Geometry check sheet. Reference: the model listing, model coordinates, mm. Face numbers are marked on the shaded views. Round coordinates to 2 decimals unless told otherwise and drop trailing zeros. Order: outer loops, then holes, each group sorted by start corner. A loop starts at its lowest first (then second) coordinate and runs counter-clockwise, first axis right, second up. Notation, with made-up numbers: (80, -7.5) - (124, -7.5) arc R29 ccw to (124, 31.5) - close; hole circle Ø7 at (17.25, 16). An arc over 180 degrees is marked (long way). Use a Markdown table: item, result. Add a question column.
(1) Mould release check, pull along Z, two halves, no side actions. Record for the marked faces 1 and 2: released by +Z, released by -Z, zero draft, split by the parting line, or undercut.
(2) Thickness scan on line 1 along Y through (x, z) = (-17, 0); line 2 along Y through (x, z) = (-42.5, 0). Record the ranges inside material, lowest first. Write a range as [from, to].
(3) Section check C-C on x = 18. Record the boundary of the cut face in (y, z), then the cut area to 3 significant figures.
(4) Section check A-A on z = 0. Record the boundary of the cut face in (x, y), then the cut area to 3 significant figures.
(5) Gauge pin test, flat ends, axial feed: P1, Ø4, axis at x = 34, y = -60.5, coming from the +Z side; P2, Ø10, axis at y = -22, z = 0, coming from the -X side; P3, Ø1, axis at y = -40, z = -28.5, coming from the -X side. Record the tip position at first contact, or that the pin passes through.
(6) Section check D-D on y = 68. Record the boundary of the cut face in (x, z).
Autodesk Inventor part; units mm, degrees
ref_plane "YZ Plane" through (0, 0, 0) normal (1, 0, 0) x (0, 1, 0)
ref_plane "XZ Plane" through (0, 0, 0) normal (0, 1, 0) x (-1, 0, 0)
ref_plane "XY Plane" through (0, 0, 0) normal (0, 0, 1) x (1, 0, 0)
sketch "Sketch1" plane through (0, 0, 0) normal (1, 0, 0) x (0, 1, 0)
  arc A0 (0, -80) -> (0, 80) centre (0, 0) ccw
  arc A1 (0, -65) -> (0, 65) centre (0, 0) ccw
  line L0 (0, 80) -> (0, 65)
  line L1 (0, -65) -> (0, -80)
  dimension "d0" = 160
  dimension "d1" = 130
revolve "Revolution1" add sketch "Sketch1" angle 180 about axis through (0, 0, 80) along (0, 0, -1)
sketch "Sketch2" plane through (0, 0, 0) normal (-1, 0, 0) x (0, 0, 1)
  circle A0 centre (0, 0) radius 80
  circle A1 centre (0, 0) radius 65
extrude "Extrusion1" add sketch "Sketch2" along normal blind 40
sketch "Sketch4" plane through (-40, 0, 0) normal (-1, 0, 0) x (0, 0, 1)
  circle A0 centre (0, 0) radius 65
  circle A1 centre (0, 0) radius 72
  dimension "d8" = 144
  dimension "d9" = 130
extrude "Extrusion3" add sketch "Sketch4" along normal blind 20
thread "Thread1"
properties part number "Bacteria Membrane Half 2"
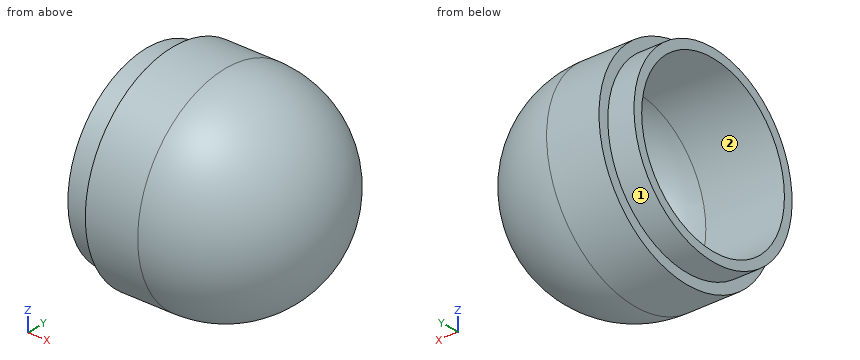
Check sheet entries:
| question | item | result |
|---|---|---|
| 1 | face 1 | split by the parting line |
| 1 | face 2 | undercut |
| 2 | line 1 | y = [-80, -65], [65, 80] |
| 2 | line 2 | y = [-72, -65], [65, 72] |
| 3 | outline | circle Ø155.9 at (0, 0); hole circle Ø124.92 at (0, 0) |
| 3 | area | 6,830 mm2 |
| 4 | outline | (-60, -72) - (-40, -72) - (-40, -80) - (0, -80) arc R80 ccw to (0, 80) - (-40, 80) - (-40, 72) - (-60, 72) - (-60, 65) - (0, 65) arc R65 cw to (0, -65) - (-60, -65) - close |
| 4 | area | 4,900 mm2 |
| 5 | P1 | stops at z = 43.1 |
| 5 | P2 | stops at x = 59.13 |
| 5 | P3 | stops at x = 41.99 |
| 6 | outline | (-60, -23.66) - (-40, -23.66) - (-40, -42.14) - (0, -42.14) arc R42.14 ccw to (0, 42.14) - (-40, 42.14) - (-40, 23.66) - (-60, 23.66) - close |
